```python
from build123d import *

# Parameters (mm, degrees)
F0_W     = 18.9141826704
F0_H     = 56.2922134995
F1_DEPTH = 12.7
F3_D     = 8.8
F5_DEPTH = 12.7
F6_SIZE  = 6.34999


# Not quite as in the source:
# - a fillet or chamfer is up to 0.001 mm smaller than in the source, because OpenCascade refuses the exact size


with BuildPart() as f1:
    # F0 (on Front) → F1 (new body)
    with BuildSketch(Plane.XZ):
        with Locations((0.1501129009, -28.1461067498)):
            Rectangle(F0_W, F0_H)
    extrude(amount=F1_DEPTH)

    # F3 (through all)
    with Locations(Plane(origin=(0, 0, 0), x_dir=(1, 0, 0), z_dir=(0, 1, 0))):
        with Locations((0, 9.7573176026), (0, 27.770826593), (0, 45.1838858426)):
            Hole(F3_D / 2)

    # F4 (on Front) → F5 (join)
    with BuildSketch(Plane.XZ):
        Polygon((0, 0), (9.6072051674, 0), (21.6162092984, 43.9829826355), (0, 73.1048211455), (-21.6162092984, 43.9829826355), (-9.6072051674, 0), align=None)
    extrude(amount=F5_DEPTH)

    # F6 (size 6.35 in the source; OpenCascade refuses exactly that, so slightly less here)
    f6_edges = [f1.edges().sort_by_distance(p)[0] for p in [
        (10.808105, 0, 58.543902),
        (-10.808105, 0, 58.543902),
        (10.808105, -12.7, 58.543902),
        (-10.808105, -12.7, 58.543902),
    ]]
    chamfer(f6_edges, length=F6_SIZE)


solid = f1.part
```
CAD build for the part. Positions are in the model's coordinates, mm. A direction names the side the tool comes from. Give positions to 0.01 mm unless a question says otherwise; leave off trailing zeros. Return JSON: item names as keys, results as strings. Group by question number.
(1) Drill centre lines: L1, parallel to Z at x = 0, y = -7; L2, parallel to Z at x = 0, y = -4.5; L3, parallel to X at y = -9, z = -5. Where is each one in solid material? Low to high. Write a range as [from, to].
(2) Band-saw the part on A-A (y = -10.5). State how many separate pieces and enclosed holes the cut face has, and give its area (3 significant figures).
(3) Flat gauge pins, fed straight in: pin 1 Ø1.5 at (y, z) = (-2, 22) entering from -X; pin 2 Ø4 at (y, z) = (-3.5, -16) entering from +X; pin 3 Ø2 at (y, z) = (-7, -32) entering from -X; pin 4 Ø10 at (x, z) = (16.5, -24.5) entering from +Y. Where does each tip first touch, or does it go through?
(4) Mould opens along X. For faces 4 (the face through (9.88, -9.57, 54.39)), 5 (the face through (0, 0, 4)), 6 (the face through (0.573, -6.439, -32.133)) say: pulls with the +X half, pulls with the -X half, needs draft (parallel to the pull), parting line crosses it, or undercut.
(5) 3-axis set-ups, long thin cutter, end or side, ignore diameter. For faces 1 (the face through (-9.307, -6, -29)), 2 (the face through (9.607, -6, -29)), 3 (the face through (0.573, -6.439, -49.546)): which of +Z, -Z, +X, -X, +Y, -Y reach the whole face in a straight line?
Entries:
{
 "1": {"L1": "z = [-56.29, -49.58], [-40.78, -32.17], [-23.37, -14.16], [-5.36, 72.01]", "L2": "z = [-56.29, -49.58], [-40.78, -32.17], [-23.37, -14.16], [-5.36, 70]", "L3": "x = [-9.31, 9.61]"},
 "2": {"separate pieces": "1", "enclosed holes": "3", "area": "2,590 mm^2"},
 "3": {"pin 1": "stops at x = -15.82", "pin 2": "stops at x = 9.61", "pin 3": "stops at x = -9.31", "pin 4": "passes through"},
 "4": {"face 4": "pulls with the +X half", "face 5": "needs draft", "face 6": "undercut"},
 "5": {"face 1": "-Z, -X, +Y, -Y", "face 2": "-Z, +X, +Y, -Y", "face 3": "+Y, -Y"}
}
